Could you check a few things on this model? Use its own coordinates, in mm. A direction names the side the tool comes from. Coordinates: 2 decimals unless noted, no trailing zeros. Order: outer loops, then holes, each group sorted by start corner. A loop starts at its lowest first (then second) coordinate and runs counter-clockwise, first axis right, second up. Notation, with made-up numbers: (-13.5, -14.5) - (14.5, -14.5) arc R21 cw to (14.5, 8.5) - close; hole circle Ø11 at (-22, 43). An arc over 180 degrees is marked (long way). One line per item, written item: value.
from build123d import *

# Parameters (mm, degrees)
F0_R     = 45.8082215722
F0_W     = 50.8
F0_H     = 50.8
F1_DEPTH = 57.15


with BuildPart() as f1:
    # F0 (on Front) → F1 (new body)
    with BuildSketch(Plane.XZ):
        with BuildLine():
            ThreePointArc((50.3805792284, -6.5143868947), (50.6950363685, -3.263937438), (50.8, 0))
            ThreePointArc((50.8, 0), (50.7758305884, 1.5668529167), (50.7033453519, 3.132214892))
            ThreePointArc((50.7033453519, 3.132214892), (36.6935912077, 35.1314725606), (5.3336979084, 50.5192207642))
            ThreePointArc((5.3336979084, 50.5192207642), (0.5040836669, 50.7974989508), (-4.3301018727, 50.6151184704))
            ThreePointArc((-4.3301018727, 50.6151184704), (-33.9875795574, 37.7555881404), (-49.88306, 9.6083466339))
            ThreePointArc((-49.88306, 9.6083466339), (-50.5702454414, 4.826), (-50.8, 0))
            ThreePointArc((-50.8, 0), (-37.7160446944, -34.0314556346), (-5.2039380863, -50.5327520366))
            ThreePointArc((-5.2039380863, -50.5327520366), (-0.3797906487, -50.7985802859), (4.4477921681, -50.6049122599))
            ThreePointArc((4.4477921681, -50.6049122599), (35.1785614294, -36.6484490225), (50.3805792284, -6.5143868947))
        make_face()
        Circle(F0_R, mode=Mode.SUBTRACT)
        Circle(F0_R)
        with Locations((1.3111739695, -1.5712582231)):
            Rectangle(F0_W, F0_H, mode=Mode.SUBTRACT)
    extrude(amount=F1_DEPTH)


solid = f1.part
Item 1: Thinking about a two-plate mould opening in X: for faces 3 (the face through (-1, 0, -33)), 4 (the face through (1, -28, 23.829)), which applies, pulls with the +X half, pulls with the -X half, needs draft (parallel to the pull), parting line crosses it, or undercut?
Conclusion:
face 3: needs draft
face 4: undercut
Item 2: I want a section at C-C on z = 20. Please give me the cut outline in (x, y).
Conclusion:
outline: (-46.7, -57.15) - (-24.09, -57.15) - (-24.09, 0) - (-46.7, 0) - close; (26.71, -57.15) - (46.7, -57.15) - (46.7, 0) - (26.71, 0) - close
Item 3: For faces 1 (the face through (-1, -57.15, -33)), 2 (the face through (26.711, -28, -2)), which set-ups out of +Z, -Z, +X, -X, +Y, -Y let a thin tool reach every point of the face, with its end or its side?
Conclusion:
face 1: +Z, -Z, +X, -X, -Y
face 2: +Y, -Y
Item 4: I want a section at D-D on x = -35.5. Please give me the cut outline in (y, z).
Conclusion:
outline: (-57.15, -36.34) - (0, -36.34) - (0, 36.34) - (-57.15, 36.34) - close
Item 5: I want a section at A-A on y = -21. Please give me the cut outline in (x, z), then the cut area to 3 significant figures.
Conclusion:
outline: circle Ø101.6 at (0, 0); hole (-24.09, -26.97) - (26.71, -26.97) - (26.71, 23.83) - (-24.09, 23.83) - close
area: 5,530 mm²
Item 6: I want a section at B-B on x = 8. Please give me the cut outline in (y, z), then the cut area to 3 significant figures.
Conclusion:
outline: (-57.15, -50.17) - (0, -50.17) - (0, -26.97) - (-57.15, -26.97) - close; (-57.15, 23.83) - (0, 23.83) - (0, 50.17) - (-57.15, 50.17) - close
area: 2,830 mm²
Item 7: If I drill on probe 1 along Z at (x, y) = (5, -31); probe 2 along X at (y, z) = (-36, 7); probe 3 along Z at (x, y) = (9, -33.5), over which ranges is the centre line in solid material (lowest first)?
Conclusion:
probe 1: -50.55 to -26.97, 23.83 to 50.55
probe 2: -50.32 to -24.09, 26.71 to 50.32
probe 3: -50 to -26.97, 23.83 to 50
Item 8: I'm going to push flat-ended pins straight in: pin 1 Ø6 at (x, y) = (-21.5, -21) entering from -Z; pin 2 Ø5 at (y, z) = (-7, -38.5) entering from +X; pin 3 Ø1.5 at (x, y) = (15.5, -40) entering from -Z. Where does each tip first touch, or does it pass through?
Conclusion:
pin 1: z = -47.31
pin 2: x = 35.84
pin 3: z = -48.61
